The listing builds one solid part. Answer for the finished solid, in the listing's coordinates (mm). A direction names the side the tool comes from. Round coordinates to 2 decimals unless told otherwise and drop trailing zeros. Write each loop counter-clockwise with the first axis right and the second up, starting at its lowest first coordinate (ties: lowest second). Pieces come first, ordered by that corner, then holes.
Item 1: Each of these flat-tipped pins is pushed along its axis until it touches: pin 1 (1.2 mm diameter, centred on x = -12, z = 18.5, fed in from +Y); pin 2 (1 mm diameter, centred on x = -1.5, y = 4.5, fed in from +Z); pin 3 (1.2 mm diameter, centred on x = 1, z = 18.5, fed in from +Y). Where does it stop, or does it pass through?
Item 2: Find section D-D on z = 0.25. Give the vertices of the cut face in (x, y), then the cut area to 3 significant figures.
Item 3: Find section C-C on x = 0. Give the vertices of the cut face in (y, z).
Item 4: A tool of negligible diameter and unlimited length cuts with its end or side. For faces 1 (the face through (14, 13, 12.49)), 2 (the face through (10.16, -7, 18)), 3 (the face through (-14, 7.62, 11)), 4 (the face through (-12, -11.811, 18)), from which of +Z, -Z, +X, -X, +Y, -Y can it reach the whole face along a straight path? Write none if from no direction.
Item 5: For a pull along X with two mould halves and no side action, classify faces 5 (the face through (-15.24, -6, 9)), 6 (the face through (12, -11, 4.572)), 7 (the face through (-14, 9, 16.764)), 8 (the face through (-11.176, -11, 4)) as +X half, -X half, draft (parallel to the pull), parting line (faces both ways), or undercut.
Item 6: Find section B-B on y = -21.5. Give the vertices of the cut face in (x, z), then the cut area to 3 significant figures.
Item 7: Find the intervals of material crossed by probe 1 along X at (y, z) = (-17.5, 3.5); probe 2 along X at (y, z) = (7.5, 1.75); probe 3 along Z at (x, y) = (1.5, -18), in increasing order.
Item 8: Find section A-A on z = 8.5. Give the vertices of the cut face in (x, y), then the cut area to 3 significant figures.
```python
from build123d import *

# Parameters (mm, degrees)
SKETCH1_W                = 30.48
SKETCH1_H                = 40.64
INITIAL_BLOCK_DEPTH      = 19.05
INITIAL_BLOCK_DEPTH_BACK = 1.778
SKETCH2_W                = 27.432
SKETCH2_H                = 19.558
INITIAL_CUT_DEPTH        = 38.1
SKETCH20_W               = 5.08
SKETCH20_H               = 10.16
SKETCH20_W_2             = 10.16
SKETCH20_H_2             = 5.08
BOSS_EXTRUDE1_DEPTH      = 1.524
SKETCH21_W               = 2.032
SKETCH21_H               = 24.13
BOSS_EXTRUDE2_DEPTH      = 2.54
SKETCH27_W               = 11.938
SKETCH27_H               = 2.032
CUT_EXTRUDE6_DEPTH       = 1.524
SKETCH28_W               = 30.48
SKETCH28_H               = 1.778
CUT_EXTRUDE7_DEPTH       = 21.828
SKETCH29_W               = 30.48
SKETCH29_H               = 2
CUT_EXTRUDE8_DEPTH       = 5.81
BOSS_EXTRUDE3_DEPTH      = 0.99
SKETCH31_W               = 30.48
SKETCH31_H               = 2.99
CUT_EXTRUDE9_DEPTH       = 0.75


with BuildPart() as part:
    # Sketch1 → Initial Block (new body, two sides)
    with BuildSketch(Plane.XY) as initial_block_sk:
        with Locations((0, -5.08)):
            Rectangle(SKETCH1_W, SKETCH1_H)
    extrude(amount=INITIAL_BLOCK_DEPTH)
    extrude(initial_block_sk.sketch, amount=-INITIAL_BLOCK_DEPTH_BACK)

    # Sketch2 → Initial Cut (cut)
    with BuildSketch(Plane(origin=(0, 15.24, 0), x_dir=(1, 0, 0), z_dir=(0, 1, 0))):
        with Locations((0, -9.271)):
            Rectangle(SKETCH2_W, SKETCH2_H)
    extrude(amount=-INITIAL_CUT_DEPTH, mode=Mode.SUBTRACT)

    # Sketch20 → Boss-Extrude1 (add)
    with BuildSketch(Plane.XY.offset(19.05)):
        with Locations((-12.7, -6.731)):
            Rectangle(SKETCH20_W, SKETCH20_H)
        with Locations((12.7, -6.731)):
            Rectangle(SKETCH20_W, SKETCH20_H)
        with Locations((0, -20.32)):
            Rectangle(SKETCH20_W_2, SKETCH20_H_2)
    extrude(amount=-BOSS_EXTRUDE1_DEPTH)

    # Sketch21 → Boss-Extrude2 (add)
    with BuildSketch(Plane(origin=(-13.716, 0, 0), x_dir=(0, 0, -1), z_dir=(1, 0, 0))):
        with Locations((-3.556, -10.795)):
            Rectangle(SKETCH21_W, SKETCH21_H)
    boss_extrude2 = extrude(amount=BOSS_EXTRUDE2_DEPTH)

    # Mirror2: Boss-Extrude2 across plane
    add(boss_extrude2.mirror(Plane(origin=(0, 0, 0), x_dir=(0, 0, 1), z_dir=(1, 0, 0))))

    # Sketch27 → Cut-Extrude6 (cut)
    with BuildSketch(Plane(origin=(15.24, 0, 0), x_dir=(0, 0, -1), z_dir=(1, 0, 0))):
        with Locations((-10.795, 8.636)):
            Rectangle(SKETCH27_W, SKETCH27_H)
    cut_extrude6 = extrude(amount=-CUT_EXTRUDE6_DEPTH, mode=Mode.SUBTRACT)

    # Mirror6: Cut-Extrude6 across plane
    add(cut_extrude6.mirror(Plane(origin=(0, 0, 0), x_dir=(0, 0, 1), z_dir=(1, 0, 0))), mode=Mode.SUBTRACT)

    # Sketch28 → Cut-Extrude7 (cut, through all)
    with BuildSketch(Plane.XY.offset(19.05)):
        with Locations((0, 14.351)):
            Rectangle(SKETCH28_W, SKETCH28_H)
    extrude(amount=-CUT_EXTRUDE7_DEPTH, mode=Mode.SUBTRACT)

    # Sketch29 → Cut-Extrude8 (cut)
    with BuildSketch(Plane.XY.offset(19.05)):
        with Locations((0, 12.462)):
            Rectangle(SKETCH29_W, SKETCH29_H)
    extrude(amount=-CUT_EXTRUDE8_DEPTH, mode=Mode.SUBTRACT)

    # Sketch30 → Boss-Extrude3 (add)
    with BuildSketch(Plane(origin=(0, 13.462, 0), x_dir=(1, 0, 0), z_dir=(0, 1, 0))):
        Polygon((-15.24, -13.24), (-15.24, 1.778), (15.24, 1.778), (15.24, -13.24), (13.716, -13.24), (13.716, 0.508), (-13.716, 0.508), (-13.716, -13.24), align=None)
    extrude(amount=BOSS_EXTRUDE3_DEPTH)

    # Sketch31 → Cut-Extrude9 (cut)
    with BuildSketch(Plane.XY.offset(13.24)):
        with Locations((0, 12.957)):
            Rectangle(SKETCH31_W, SKETCH31_H)
    extrude(amount=-CUT_EXTRUDE9_DEPTH, mode=Mode.SUBTRACT)


solid = part.part
```
Check values:
1. pin 1: stops at y = -1.65
1. pin 2: stops at z = -0.51
1. pin 3: stops at y = -17.78
2. outline: (-15.24, -25.4) - (15.24, -25.4) - (15.24, 14.45) - (13.72, 14.45) - (13.72, -22.86) - (-13.72, -22.86) - (-13.72, 14.45) - (-15.24, 14.45) - close
2. area: 191 mm2
3. outline: (-25.4, -1.78) - (14.45, -1.78) - (14.45, -0.51) - (-22.86, -0.51) - (-22.86, 17.53) - (-17.78, 17.53) - (-17.78, 19.05) - (-25.4, 19.05) - close
4. face 1: +Z, +X, -X, +Y
4. face 2: +Z, +Y
4. face 3: +X, -X
4. face 4: +Z
5. face 5: -X half
5. face 6: undercut
5. face 7: draft
5. face 8: undercut
6. outline: (-15.24, -1.78) - (15.24, -1.78) - (15.24, 19.05) - (13.72, 19.05) - (13.72, 4.57) - (11.18, 4.57) - (11.18, 2.54) - (13.72, 2.54) - (13.72, -0.51) - (-13.72, -0.51) - (-13.72, 2.54) - (-11.18, 2.54) - (-11.18, 4.57) - (-13.72, 4.57) - (-13.72, 19.05) - (-15.24, 19.05) - close; (-5.08, 17.53) - (5.08, 17.53) - (5.08, 19.05) - (-5.08, 19.05) - close
6. area: 124 mm2
7. probe 1: x = -15.24 to -11.18, 11.18 to 15.24
7. probe 2: x = -15.24 to -13.72, 13.72 to 15.24
7. probe 3: z = -1.78 to -0.51, 17.53 to 19.05
8. outline: (-15.24, -25.4) - (15.24, -25.4) - (15.24, 7.62) - (13.72, 7.62) - (13.72, -22.86) - (-13.72, -22.86) - (-13.72, 7.62) - (-15.24, 7.62) - close; (-15.24, 9.65) - (-13.72, 9.65) - (-13.72, 14.45) - (-15.24, 14.45) - close; (13.72, 9.65) - (15.24, 9.65) - (15.24, 14.45) - (13.72, 14.45) - close
8. area: 185 mm2
